from build123d import *

# Parameters (mm, degrees)
F0_W      = 24
F0_H      = 18
F2_DEPTH  = 8.5
F1_W      = 20
F1_H      = 12
F1_R      = 1.25
F3_DEPTH  = 6.5
F4_R      = 1
F5_DEPTH  = 25
F3_FACE_W = 20
F3_FACE_H = 6.5
F6_DEPTH  = 4.5


with BuildPart() as f2:
    # F0 (on Top) → F2 (new body)
    with BuildSketch(Plane.XY):
        with Locations((0, 3)):
            Rectangle(F0_W, F0_H)
    extrude(amount=F2_DEPTH)

    # F1 (on Top) → F3 (cut)
    with BuildSketch(Plane.XY):
        Rectangle(F1_W, F1_H)
        with Locations((-4.5, -3)):
            Circle(F1_R, mode=Mode.SUBTRACT)
        with Locations((4.5, -3)):
            Circle(F1_R, mode=Mode.SUBTRACT)
    extrude(amount=F3_DEPTH, mode=Mode.SUBTRACT)

    # F4 (on face) → F5 (cut)
    with BuildSketch(Plane(origin=(-12, 0, 0), x_dir=(0, -1, 0), z_dir=(-1, 0, 0))):
        with Locations((-9, 4.276814)):
            Circle(F4_R)
    extrude(amount=-F5_DEPTH, mode=Mode.SUBTRACT)

    # F3_face (on face) → F6 (cut)
    with BuildSketch(Plane(origin=(0, 6, 3.25), x_dir=(1, 0, 0), z_dir=(0, -1, 0))):
        Rectangle(F3_FACE_W, F3_FACE_H)
    extrude(amount=-F6_DEPTH, mode=Mode.SUBTRACT)


solid = f2.part
For this review, take the finished solid that the model builds, in its own axes (mm). A direction names the side the tool comes from. Give positions to 0.01 mm unless a question says otherwise; leave off trailing zeros. Loops run counter-clockwise (first coordinate to the right, second up) from the corner with the lowest first, then second, coordinate; pieces in that order, holes last. Notation, with made-up numbers: M 62,25 L 116,25 A28 ccw 116,43 Z; hole C 70.25,-5 d6. An arc over 180 degrees is marked long. Answer as a JSON object with one key per item and string values. Group by question number.
Q1. Add section D-D on x = 4.5. Give the boundary of the cut face in (y, z), and give its area (3 significant figures).
Q2. Add section C-C on y = -2.25. Give the boundary of the cut face in (x, z).
Q3. Tool access review of faces 1 (the cylindrical face through (-11.014, 9.794, 3.668)), 2 (the cylindrical face through (-5.421, -2.155, 3.204)), 3 (the flat face through (10, 2, 3)): name each direction out of +Z, -Z, +X, -X, +Y, -Y from which nothing blocks a thin tool from reaching the whole face with its end or side.
Q4. Insertion check: P1, Ø5, axis at x = -1, z = 3.5, coming from the -Y side; P2, Ø2, axis at x = 8, y = -2, coming from the -Z side. Each pin has a flat end and moves straight along its axis. Give the tip position at first contact, or say it passes through.
Q5. Mouldability with a two-part tool opening along Y and no side actions: class faces 4 (the cylindrical face through (3.579, -2.155, 3.204)), 5 (the flat face through (0, -6, 7)), 6 (the flat face through (-2, 11, 0)) as +Y half, -Y half, draft (parallel to the pull), parting line (faces both ways), or undercut.
Q6. Add section A-A on z = 6. Give the boundary of the cut face in (x, y), and give its area (3 significant figures).
Q7. For probe 1 along Z at (x, y) = (-11.35, 9); probe 2 along X at (y, z) = (-5, 4.5); probe 3 along Z at (x, y) = (4.5, 9.5), list the stretches that pass through material, from the lowest coordinate up. Write a range as [from, to].
Q8. Add section B-B on y = 9. Give the boundary of the cut face in (x, z), and give its area (3 significant figures).
Checked values:
{
 "1": {"outline": "M -6,6.5 L -4.25,6.5 L -4.25,0 L -1.75,0 L -1.75,6.5 L 10.5,6.5 L 10.5,0 L 12,0 L 12,8.5 L -6,8.5 Z", "area": "62.0 mm²"},
 "2": {"outline": "M -12,0 L -10,0 L -10,6.5 L -5.5,6.5 L -5.5,0 L -3.5,0 L -3.5,6.5 L 3.5,6.5 L 3.5,0 L 5.5,0 L 5.5,6.5 L 10,6.5 L 10,0 L 12,0 L 12,8.5 L -12,8.5 Z"},
 "3": {"face 1": "+X, -X", "face 2": "-Z", "face 3": "-Z, -Y"},
 "4": {"P1": "y = -3.75", "P2": "z = 6.5"},
 "5": {"face 4": "undercut", "face 5": "-Y half", "face 6": "draft"},
 "6": {"outline": "M -12,-6 L -10,-6 L -10,10.5 L 10,10.5 L 10,-6 L 12,-6 L 12,12 L -12,12 Z; C -4.5,-3 d2.5; C 4.5,-3 d2.5", "area": "112 mm²"},
 "7": {"probe 1": "[0, 3.28], [5.28, 8.5]", "probe 2": "[-12, -10], [10, 12]", "probe 3": "[6.5, 8.5]"},
 "8": {"outline": "M -12,0 L -10,0 L -10,3.28 L -12,3.28 Z; M -12,5.28 L -10,5.28 L -10,6.5 L 10,6.5 L 10,5.28 L 12,5.28 L 12,8.5 L -12,8.5 Z; M 10,0 L 12,0 L 12,3.28 L 10,3.28 Z", "area": "66.0 mm²"}
}
